```python
from build123d import *

# Parameters (mm, degrees)
SKETCH3_OUTSIDE_W = 46.516
SKETCH3_OUTSIDE_H = 46.516
HEX_2_DEPTH       = 26.740629363
INNERCHAMFER_SIZE = 0.38


with BuildPart() as part:
    # Sketch2 → Body (revolve)
    with BuildSketch(Plane(origin=(0, 0, 0), x_dir=(0, 0, -1), z_dir=(1, 0, 0)), mode=Mode.PRIVATE) as body_sk:
        Polygon((-4, 9.5), (-4, 15), (-2.672094381, 17.3), (2.672094381, 17.3), (4, 15), (4, 9.5), align=None)
    revolve(body_sk.sketch.rotate(Axis((0, 0, 27.389186195), (0, 0, 1)), 90), axis=Axis((0, 0, 27.389186195), (0, 0, 1)))

    # Sketch3 outside → Hex 2 (cut, through all)
    with BuildSketch(Plane.XY.offset(4)):
        Rectangle(SKETCH3_OUTSIDE_W, SKETCH3_OUTSIDE_H)
        Polygon((14.982239485, -8.65), (14.982239485, 8.65), (0, 17.3), (-14.982239485, 8.65), (-14.982239485, -8.65), (0, -17.3), align=None, mode=Mode.SUBTRACT)
    extrude(amount=-HEX_2_DEPTH, mode=Mode.SUBTRACT)

    # InnerChamfer
    innerchamfer_edges = [part.edges().sort_by_distance(p)[0] for p in [
        (9.5, 0, 4),
        (9.5, 0, -4),
    ]]
    chamfer(innerchamfer_edges, length=INNERCHAMFER_SIZE)


solid = part.part
```
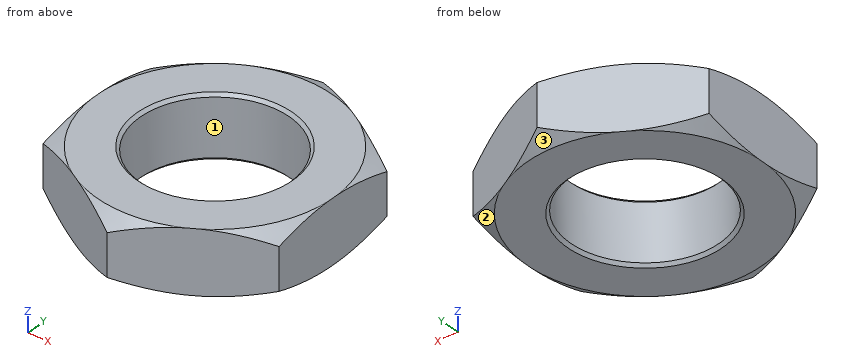
Read the model definition and answer for the solid it produces. Units are mm, in the model's axes. Face numbers are marked on the shaded views. Coordinates: 2 decimals unless noted, no trailing zeros. Loops run counter-clockwise (first coordinate to the right, second up) from the corner with the lowest first, then second, coordinate; pieces in that order, holes last. Notation, with made-up numbers: (60, 9) - (117, 9) arc R21 ccw to (117, 24) - close; hole circle Ø4 at (-9, 55). An arc over 180 degrees is marked (long way). Answer in a Markdown table with one row per item.
1. Given pin 1 (6 mm diameter, centred on x = 9, y = -12.5, fed in from -Z); pin 2 (2 mm diameter, centred on y = 12.5, z = 2, fed in from +X), each flat-ended and moving along its own axis, determine where each tip first touches the part or whether it passes through.
Conclusion:
| item | result |
|---|---|
| pin 1 | stops at z = -4 |
| pin 2 | stops at x = 10.05 |
2. Straight lines are drawn through the part: line 1 (Y direction, x = 0, z = 3); line 2 (Y direction, x = -5.25, z = -0.75); line 3 (X direction, y = 8.5, z = 1.75). For each, find the intervals that lie inside material, in ascending order.
Conclusion:
| item | result |
|---|---|
| line 1 | y = -16.73 to -9.5, 9.5 to 16.73 |
| line 2 | y = -14.27 to -7.92, 7.92 to 14.27 |
| line 3 | x = -14.98 to -4.24, 4.24 to 14.98 |
3. Determine the mould class of the marked faces 1, 2 and 3 for opening direction X: +X half, -X half, draft (parallel to the pull), parting line (faces both ways), or undercut.
Conclusion:
| item | result |
|---|---|
| face 1 | undercut |
| face 2 | +X half |
| face 3 | parting line |
4. Find section A-A, the plane z = 0. Write down the section's boundary in (x, y).
Conclusion:
| item | result |
|---|---|
| outline | (-14.98, -8.65) - (0, -17.3) - (14.98, -8.65) - (14.98, 8.65) - (0, 17.3) - (-14.98, 8.65) - close; hole circle Ø19 at (0, 0) |
